from build123d import *

# Parameters (mm, degrees)
SZKIC1_W                                          = 237
SZKIC1_H                                          = 150
DODANIE_WYCI_GNI_CIE1_DEPTH                       = 5
SZKIC2_W                                          = 7
SZKIC2_H                                          = 135
DODANIE_WYCI_GNI_CIE2_DEPTH                       = 10
OTW_R_4_0_4_1_D                                   = 4
OTW_R_4_0_4_1_DEPTH                               = 6.7
SFAZOWANIE1_SIZE                                  = 10
POG_BIENIE_WALCOWE_POD_M3_RUB_Z_BEM_S_D           = 3.6
POG_BIENIE_WALCOWE_POD_M3_RUB_Z_BEM_S_DEPTH       = 6.7
POG_BIENIE_WALCOWE_POD_M3_RUB_Z_BEM_S_CBORE_D     = 7
POG_BIENIE_WALCOWE_POD_M3_RUB_Z_BEM_S_CBORE_DEPTH = 2.4
POG_BIENIE_WALCOWE_POD_M3_RUB_Z_BEM_S_TIP         = 1.081549114
OTWORY_USTALAJ_CE_4_0MM1_D                        = 4
OTWORY_USTALAJ_CE_4_0MM1_DEPTH                    = 6.7


with BuildPart() as part:
    # Szkic1 → Dodanie-wyciągnięcie1 (new body)
    with BuildSketch(Plane.XY):
        Rectangle(SZKIC1_W, SZKIC1_H)
    extrude(amount=DODANIE_WYCI_GNI_CIE1_DEPTH)

    # Szkic2 → Dodanie-wyciągnięcie2 (add)
    with BuildSketch(Plane.XY.offset(5)):
        with Locations((115, -2.5)):
            Rectangle(SZKIC2_W, SZKIC2_H)
        with Locations((-115, -2.5)):
            Rectangle(SZKIC2_W, SZKIC2_H)
    extrude(amount=DODANIE_WYCI_GNI_CIE2_DEPTH)

    # Otwór Ø4.0 (4)1
    with Locations(Plane(origin=(118.5, 0, 0), x_dir=(0, 0, -1), z_dir=(1, 0, 0))):
        with Locations((-10, -37.5), (-10, 37.5), (-10, 0)):
            otw_r_4_0_4_1 = Hole(OTW_R_4_0_4_1_D / 2, depth=OTW_R_4_0_4_1_DEPTH)

    # Lustro1: Otwór Ø4.0 (4)1 across plane
    add(otw_r_4_0_4_1.mirror(Plane.ZY), mode=Mode.SUBTRACT)

    # Sfazowanie1
    sfazowanie1_edges = [part.edges().sort_by_distance(p)[0] for p in [
        (-115, 65, 15),
        (115, 65, 15),
    ]]
    chamfer(sfazowanie1_edges, length=SFAZOWANIE1_SIZE - 0.0001)  # a hair under: the kernel refuses the full size

    # Pogłębienie walcowe pod M3 Śrubę z łbem stożkowym ściętym1
    with Locations(Plane(origin=(0, 0, 0), x_dir=(-1, 0, 0), z_dir=(0, 0, -1))):
        with Locations((-79, 70), (-39.5, 70), (79, 70), (0, 70), (39.5, 70)):
            CounterBoreHole(POG_BIENIE_WALCOWE_POD_M3_RUB_Z_BEM_S_D / 2, POG_BIENIE_WALCOWE_POD_M3_RUB_Z_BEM_S_CBORE_D / 2, POG_BIENIE_WALCOWE_POD_M3_RUB_Z_BEM_S_CBORE_DEPTH, depth=POG_BIENIE_WALCOWE_POD_M3_RUB_Z_BEM_S_DEPTH)
            with Locations((0, 0, -(POG_BIENIE_WALCOWE_POD_M3_RUB_Z_BEM_S_DEPTH + POG_BIENIE_WALCOWE_POD_M3_RUB_Z_BEM_S_TIP / 2))):  # 118° drill point
                Cone(0, POG_BIENIE_WALCOWE_POD_M3_RUB_Z_BEM_S_D / 2, POG_BIENIE_WALCOWE_POD_M3_RUB_Z_BEM_S_TIP, mode=Mode.SUBTRACT)

    # Otwory ustalające Ø4.0mm1
    with Locations(Plane.XZ.offset(70)):
        with Locations((115, 10), (-115, 10)):
            Hole(OTWORY_USTALAJ_CE_4_0MM1_D / 2, depth=OTWORY_USTALAJ_CE_4_0MM1_DEPTH)


solid = part.part
For this review, take the finished solid that the model builds, in its own axes (mm). A direction names the side the tool comes from. Round coordinates to 2 decimals unless told otherwise and drop trailing zeros. Order: outer loops, then holes, each group sorted by start corner. A loop starts at its lowest first (then second) coordinate and runs counter-clockwise, first axis right, second up. Notation, with made-up numbers: M 69.25,-36.75 L 94.25,-36.75 A15 cw 94.25,-9.75 Z; hole C -5.75,-6.75 d8. An arc over 180 degrees is marked long. Use a Markdown table: item, result. Add a question column.
Item 1: Insertion check: pin 1 (3.5 mm diameter, centred on y = -37.5, z = 10, fed in from -X); pin 2 (2 mm diameter, centred on x = -114.5, z = 10.5, fed in from -Y); pin 3 (2 mm diameter, centred on x = -38.5, y = 71.5, fed in from -Z). Each pin has a flat end and moves straight along its axis. Give the tip position at first contact, or say it passes through.
Item 2: Mouldability with a two-part tool opening along Y and no side actions: class faces 1 (the flat face through (-118.5, -1, 7)), 2 (the flat face through (-2, 75, 2)), 3 (the flat face through (40, 72, 2.4)) as released by +Y, released by -Y, zero draft, split by the parting line, or undercut.
Item 3: To check wall thickness, follow line 1 along Y through (x, z) = (0, 1.3); line 2 along Y through (x, z) = (-79, 3.45); line 3 along X through (y, z) = (59.5, 9.5). State the ranges of each line that lie inside material, in increasing order.
Item 4: Add section A-A, the plane y = -51.5. Give the boundary of the cut face in (x, z).
Item 5: Add section B-B, the plane x = -89.5. Give the boundary of the cut face in (y, z).
Item 6: Tool access review of faces 4 (the cylindrical face through (-36.7, 67.9, 1.2)), 5 (the flat face through (-115, -70, 12.2)), 6 (the flat face through (-111.5, -3, 10)), 7 (the flat face through (-115, 60, 10)): name each direction out of +Z, -Z, +X, -X, +Y, -Y from which nothing blocks a thin tool from reaching the whole face with its end or side.
Geometry results:
| question | item | result |
|---|---|---|
| 1 | pin 1 | stops at x = -111.8 |
| 1 | pin 2 | stops at y = -63.3 |
| 1 | pin 3 | stops at z = 2.4 |
| 2 | face 1 | zero draft |
| 2 | face 2 | released by +Y |
| 2 | face 3 | undercut |
| 3 | line 1 | y = -75 to 66.5, 73.5 to 75 |
| 3 | line 2 | y = -75 to 68.2, 71.8 to 75 |
| 3 | line 3 | x = -118.5 to -111.5, 111.5 to 118.5 |
| 4 | outline | M -118.5,0 L 118.5,0 L 118.5,15 L 111.5,15 L 111.5,5 L -111.5,5 L -111.5,15 L -118.5,15 Z |
| 5 | outline | M -75,0 L 75,0 L 75,5 L -75,5 Z |
| 6 | face 4 | -Z |
| 6 | face 5 | +Z, +X, -X, -Y |
| 6 | face 6 | +Z, +Y, -Y |
| 6 | face 7 | +Z, +X, -X, +Y |
